Drawing for the job (mm, zero at the part's lowest x, y, z). A direction names the side the tool comes from. Coordinates: 2 decimals unless noted, no trailing zeros. Write each loop counter-clockwise with the first axis right and the second up, starting at its lowest first coordinate (ties: lowest second). Pieces come first, ordered by that corner, then holes. Notation, with made-up numbers: M 87,-8 L 142,-8 A26 cw 142,16 Z; hole C 13,-38 d2. An arc over 180 degrees is marked long. Use a Markdown table: item, result. Add a question column.
Q1. Slice it at C-C on x = 28.25. Write the cut outline in (y, z), then the cut area to 3 significant figures.
Q2. Slice it at D-D on y = 6. Write the cut outline in (x, z), then the cut area to 3 significant figures.
Q3. Slice it at A-A on y = 24. Write the cut outline in (x, z).
Q4. Slice it at B-B on z = 25. Write the cut outline in (x, y).
Q5. Tool access for the marked faces 1 and 2: list every direction of +Z, -Z, +X, -X, +Y, -Y with a clear straight run to the whole face (end or side of a thin tool).
Q6. Mould opens along Z. For the marked faces 3, 4 and 5 say: released by +Z, released by -Z, zero draft, split by the parting line, or undercut.
Q7. Pin check, flat tips, straight feed: pin 1 Ø8 at (x, z) = (127.5, 42.5) entering from +Y; pin 2 Ø12 at (y, z) = (46.5, 15.5) entering from -X; pin 3 Ø19 at (x, z) = (97, 25) entering from +Y; pin 4 Ø10 at (x, z) = (50.5, 37.5) entering from -Y. Stop position of each tip, or through.
Q8. Wall check: L1, parallel to X at y = 47.75, z = 25; L2, parallel to X at y = 7.5, z = 25; L3, parallel to X at y = 33, z = 23. Give the ranges that are in metal, low to high. Write a range as from..to.
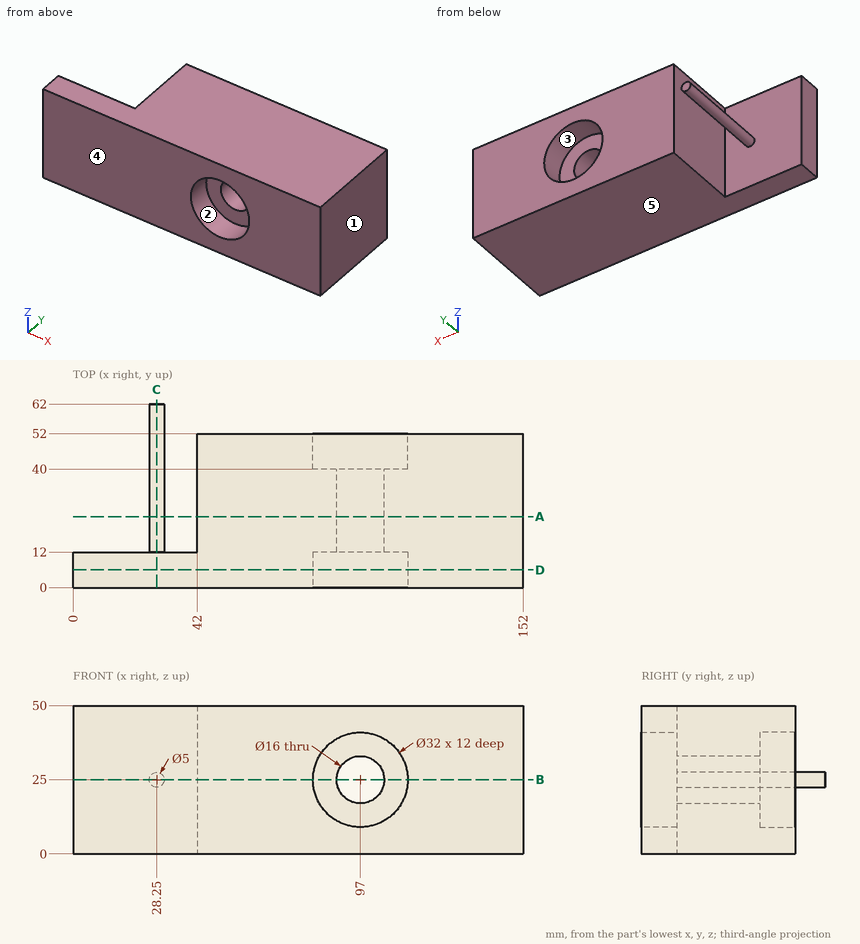
Recorded:
| question | item | result |
|---|---|---|
| 1 | outline | M 0,0 L 12,0 L 12,22.5 L 62,22.5 L 62,27.5 L 12,27.5 L 12,50 L 0,50 Z |
| 1 | area | 850 mm² |
| 2 | outline | M 0,0 L 152,0 L 152,50 L 0,50 Z; hole C 97,25 d32 |
| 2 | area | 6,800 mm² |
| 3 | outline | C 28.25,25 d5; M 42,0 L 152,0 L 152,50 L 42,50 Z; hole C 97,25 d16 |
| 4 | outline | M 0,0 L 81,0 L 81,12 L 89,12 L 89,40 L 81,40 L 81,52 L 42,52 L 42,12 L 30.75,12 L 30.75,62 L 25.75,62 L 25.75,12 L 0,12 Z; M 105,12 L 113,12 L 113,0 L 152,0 L 152,52 L 113,52 L 113,40 L 105,40 Z |
| 5 | face 1 | +Z, -Z, +X, +Y, -Y |
| 5 | face 2 | -Y |
| 6 | face 3 | undercut |
| 6 | face 4 | zero draft |
| 6 | face 5 | released by -Z |
| 7 | pin 1 | y = 52 |
| 7 | pin 2 | x = 42 |
| 7 | pin 3 | y = 40 |
| 7 | pin 4 | y = 0 |
| 8 | L1 | 25.75..30.75, 42..81, 113..152 |
| 8 | L2 | 0..81, 113..152 |
| 8 | L3 | 26.75..29.75, 42..89.25, 104.75..152 |
